Input: dimensioned drawing with shaded views. Units: mm. Origin: part minimum x, y, z. A direction names the side the tool comes from. Give positions to 0.01 mm unless a question says otherwise; leave off trailing zeros. Write each loop counter-clockwise with the first axis right and the second up, starting at its lowest first coordinate (ties: lowest second). Pieces come first, ordered by that corner, then holes. Notation, with made-up numbers: (-15, 71.25) -> (-7, 71.25) arc R16 cw to (-7, 76.25) -> close; hole circle Ø9 at (37, 75.25). An arc over 180 degrees is marked (long way). Answer in a Markdown table with one row per item. Add a question column.
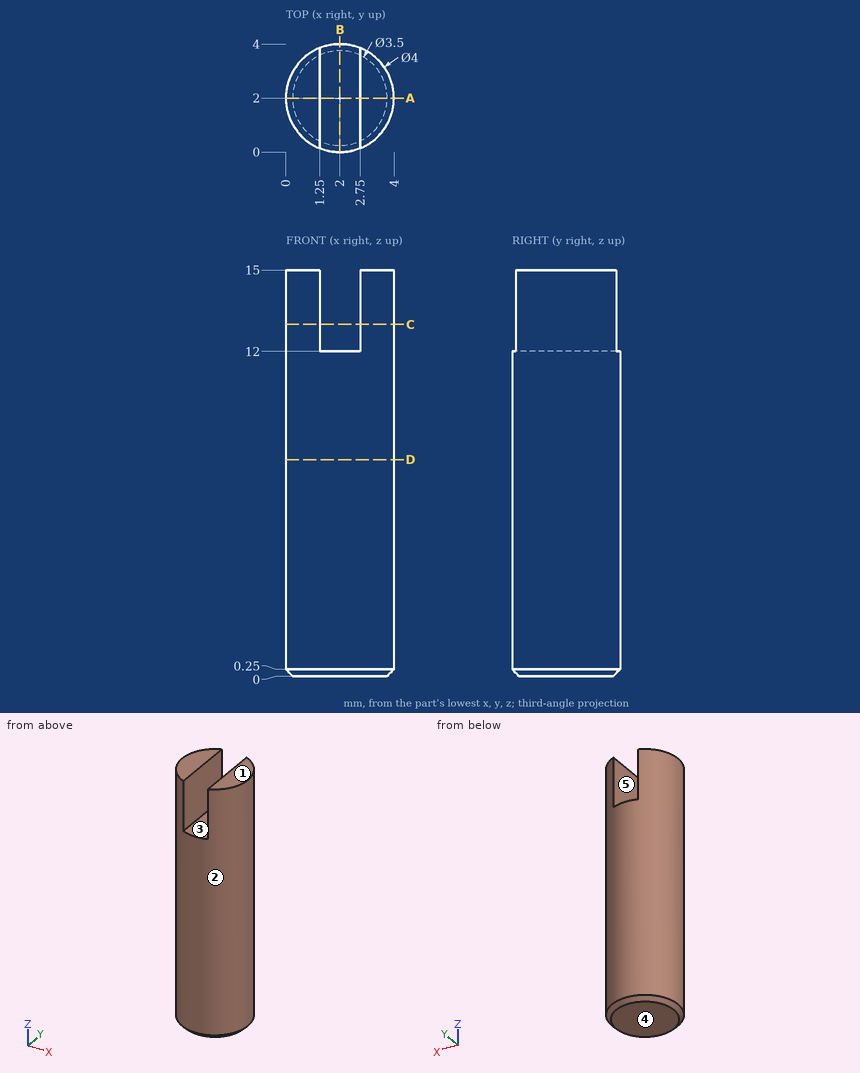
Q1. Section A-A on y = 2. Return loops of the section in (x, z), and give its area (3 significant figures).
Q2. Access query for the marked faces 4 and 5. Directions: +Z, -Z, +X, -X, +Y, -Y. A direction counts if a zero-diameter tool reaches every point of the face in a straight line with its end or side. Return the directions, or none.
Q3. Line query: probe 1 along X at (y, z) = (2.6, 13); probe 2 along Z at (x, y) = (2.3, 2.95); probe 3 along X at (y, z) = (2.8, 12.75). Output: solid intervals per line, ascending. Write a range as from..to.
Q4. Section B-B on x = 2. Return loops of the section in (y, z).
Q5. Section C-C on z = 13. Return loops of the section in (x, y), and give its area (3 significant figures).
Q6. Contact query for flat-ended pins moving along their axis: pin 1 Ø1.5 at (y, z) = (2.5, 8) entering from -X; pin 2 Ø0.8 at (x, y) = (2, 3) entering from +Z; pin 3 Ø1 at (y, z) = (0.5, 12.5) entering from -X. Output: stop coordinate, or through.
Q7. Pull-direction query (X, two-part tool) for the marked faces 1, 2 and 3; classes: +X half, -X half, draft (parallel to the pull), parting line (faces both ways), or undercut.
Q8. Section D-D on z = 8. Return loops of the section in (x, y).
Checks:
| question | item | result |
|---|---|---|
| 1 | outline | (0, 0.25) -> (0.25, 0) -> (3.75, 0) -> (4, 0.25) -> (4, 15) -> (2.75, 15) -> (2.75, 12) -> (1.25, 12) -> (1.25, 15) -> (0, 15) -> close |
| 1 | area | 55.4 mm^2 |
| 2 | face 4 | -Z, +X, -X, +Y, -Y |
| 2 | face 5 | +Z, +Y, -Y |
| 3 | probe 1 | 0.09..1.25, 2.75..3.91 |
| 3 | probe 2 | 0..12 |
| 3 | probe 3 | 0.17..1.25, 2.75..3.83 |
| 4 | outline | (0, 0.25) -> (0.25, 0) -> (3.75, 0) -> (4, 0.25) -> (4, 12) -> (0, 12) -> close |
| 5 | outline | (1.25, 0.15) -> (1.25, 3.85) arc R2 ccw to start; (2.75, 0.15) arc R2 ccw to (2.75, 3.85) -> close |
| 5 | area | 6.71 mm^2 |
| 6 | pin 1 | x = 0 |
| 6 | pin 2 | z = 12 |
| 6 | pin 3 | x = 0.27 |
| 7 | face 1 | draft |
| 7 | face 2 | parting line |
| 7 | face 3 | undercut |
| 8 | outline | circle Ø4 at (2, 2) |
